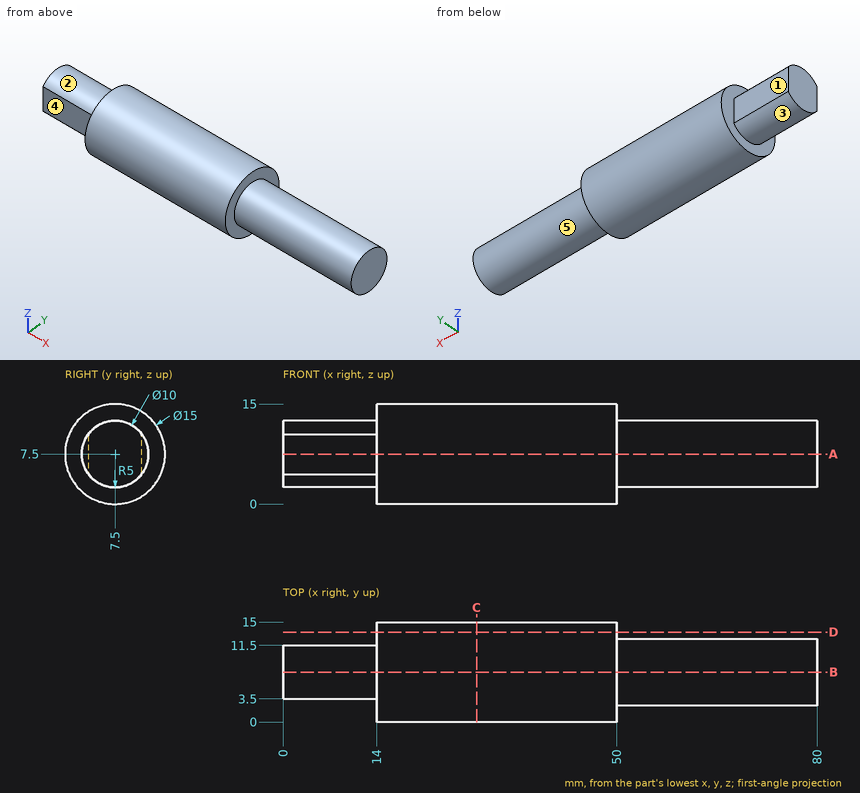
Verification items for this drawing (mm, ordinates from the low corner). A direction names the side the tool comes from. Give positions to 0.01 mm unless a question says otherwise; leave off trailing zeros. Loops run counter-clockwise (first coordinate to the right, second up) from the corner with the lowest first, then second, coordinate; pieces in that order, holes last. Notation, with made-up numbers: M -11,69 L -4,69 A24 ccw -4,102 Z; hole C 80,83.5 d10. An arc over 180 degrees is marked long. Return JSON: item names as keys, results as strings. Group by question number.
1. Cross-section at B-B on y = 7.5. Record the boundary of the cut face in (x, z).
2. Go/stop test with flat-tipped pins: pin 1 (1.5 mm diameter, centred on x = 57, z = 8.5, fed in from +Y); pin 2 (5 mm diameter, centred on x = 8, z = 7, fed in from +Y); pin 3 (5 mm diameter, centred on x = 4, z = 7, fed in from -Y). Record where each tip stops, or that it passes through.
3. Thickness scan on L1, parallel to X at y = 9.25, z = 1.5; L2, parallel to Y at x = 77, z = 4.5. Record the ranges inside material, lowest first.
4. Cross-section at C-C on x = 29. Record the boundary of the cut face in (y, z).
5. Cross-section at A-A on z = 7.5. Record the boundary of the cut face in (x, y).
6. Cross-section at D-D on y = 13.5. Record the boundary of the cut face in (x, z), plus the area to 3 significant figures.
7. Tool access check on the marked faces 1, 2, 3, 4 and 5. Record the directions out of +Z, -Z, +X, -X, +Y, -Y that give a thin tool (end or side, any length) a straight path to the whole face; none if there is none.
Return value:
{
 "1": {"outline": "M 0,2.5 L 14,2.5 L 14,0 L 50,0 L 50,2.5 L 80,2.5 L 80,12.5 L 50,12.5 L 50,15 L 14,15 L 14,12.5 L 0,12.5 Z"},
 "2": {"pin 1": "y = 12.49", "pin 2": "y = 11.5", "pin 3": "y = 3.5"},
 "3": {"L1": "14 to 50", "L2": "3.5 to 11.5"},
 "4": {"outline": "C 7.5,7.5 d15"},
 "5": {"outline": "M 0,3.5 L 14,3.5 L 14,0 L 50,0 L 50,2.5 L 80,2.5 L 80,12.5 L 50,12.5 L 50,15 L 14,15 L 14,11.5 L 0,11.5 Z"},
 "6": {"outline": "M 14,3 L 50,3 L 50,12 L 14,12 Z", "area": "324 mm^2"},
 "7": {"face 1": "+Z, -Z, -X, +Y", "face 2": "+Z, -X", "face 3": "-Z, -X", "face 4": "+Z, -Z, -X, -Y", "face 5": "+X"}
}
